Can you work these out from the model? Positions are in its coordinate system, mm. Coordinates: 2 decimals unless noted, no trailing zeros. Order: outer loops, then holes, each group sorted by start corner. A loop starts at its lowest first (then second) coordinate and runs counter-clockwise, first axis right, second up.
```python
from build123d import *

# Parameters (mm, degrees)
SKETCH1_W          = 100
SKETCH1_H          = 120
SKETCH1_R          = 3.25
BASE_FLANGE1_DEPTH = 5
FILLET1_R          = 5


# Sheet-metal steps are written as plain solids
with BuildPart() as part:
    # Sketch1 → Base-Flange1 (new body)
    with BuildSketch(Plane.XY):
        Rectangle(SKETCH1_W, SKETCH1_H)
        with Locations((-27.5, 30)):
            Circle(SKETCH1_R, mode=Mode.SUBTRACT)
        with Locations((27.5, 30)):
            Circle(SKETCH1_R, mode=Mode.SUBTRACT)
        with Locations((-27.5, -35)):
            Circle(SKETCH1_R, mode=Mode.SUBTRACT)
        with Locations((27.5, -35)):
            Circle(SKETCH1_R, mode=Mode.SUBTRACT)
    extrude(amount=-BASE_FLANGE1_DEPTH)

    # Fillet1
    fillet1_edges = [part.edges().sort_by_distance(p)[0] for p in [
        (50, -60, -2.5),
        (-50, -60, -2.5),
        (-50, 60, -2.5),
        (50, 60, -2.5),
    ]]
    fillet(fillet1_edges, radius=FILLET1_R)


solid = part.part
```
1. Thinking about a two-plate mould opening in Y: for faces 1 (the flat face through (50, -1, -2)), 2 (the cylindrical face through (-49, 58, -3)), 3 (the cylindrical face through (48, -59, -3)), 4 (the cylindrical face through (29, 27.117, -2.465)), which applies, pulls with the +Y half, pulls with the -Y half, needs draft (parallel to the pull), parting line crosses it, or undercut?
Completed:
face 1: needs draft
face 2: pulls with the +Y half
face 3: pulls with the -Y half
face 4: undercut
2. I'm going to push a flat-ended pin straight in: pin 1 (7.5 mm diameter, centred on x = -27.5, y = 30, fed in from +Z). Where does the tip first touch, or does it pass through?
Completed:
pin 1: stops at z = 0
3. Imagine slicing it at A-A on y = -35. Please give me the cut outline in (x, z).
Completed:
outline: (-50, -5) - (-30.75, -5) - (-30.75, 0) - (-50, 0) - close; (-24.25, -5) - (24.25, -5) - (24.25, 0) - (-24.25, 0) - close; (30.75, -5) - (50, -5) - (50, 0) - (30.75, 0) - close
4. Imagine slicing it at B-B on x = 27.5. Please give me the cut outline in (y, z), then the cut area to 3 significant figures.
Completed:
outline: (-60, -5) - (-38.25, -5) - (-38.25, 0) - (-60, 0) - close; (-31.75, -5) - (26.75, -5) - (26.75, 0) - (-31.75, 0) - close; (33.25, -5) - (60, -5) - (60, 0) - (33.25, 0) - close
area: 535 mm2
5. Please list where these lines run through material, in increasing order: probe 1 along Y at (x, z) = (27.5, -2.2); probe 2 along X at (y, z) = (-33, -3.85); probe 3 along Y at (x, z) = (-24.5, -4.45).
Completed:
probe 1: y = -60 to -38.25, -31.75 to 26.75, 33.25 to 60
probe 2: x = -50 to -30.06, -24.94 to 24.94, 30.06 to 50
probe 3: y = -60 to -36.25, -33.75 to 28.75, 31.25 to 60
